The listing builds one solid part. Answer for the finished solid, in the listing's coordinates (mm). Coordinates: 2 decimals unless noted, no trailing zeros. Loops run counter-clockwise (first coordinate to the right, second up) from the corner with the lowest first, then second, coordinate; pieces in that order, holes last. Notation, with made-up numbers: (-38.75, 50) - (9.25, 50) arc R23 cw to (9.25, 89) - close; hole circle Ø6 at (42.5, 43). An arc over 180 degrees is marked (long way). Put each result on its own line as item: value.
```python
from build123d import *

# Parameters (mm, degrees)
F0_R     = 6.35
F0_R_2   = 3.81
F1_DEPTH = 7.62


with BuildPart() as f1:
    # F0 (on Front) → F1 (new body)
    with BuildSketch(Plane.XZ):
        with BuildLine():
            ThreePointArc((-8.547501, -17.972921), (0, -26.520421), (8.547501, -17.972921))
            Line((8.547501, -17.972921), (5.813845, 25.207079))
            ThreePointArc((5.813845, 25.207079), (0, 31.020925), (-5.813845, 25.207079))
            Line((-5.813845, 25.207079), (-8.547501, -17.972921))
        make_face()
        with Locations((0, -17.972921)):
            Circle(F0_R, mode=Mode.SUBTRACT)
        with Locations((0, 25.207079)):
            Circle(F0_R_2, mode=Mode.SUBTRACT)
    extrude(amount=F1_DEPTH)


solid = f1.part
```
1) For a pull along X with two mould halves and no side action, classify faces 1 (the face through (0, -7.62, 3)), 2 (the face through (7.2, -3.8, 3.3)), 3 (the face through (-1.38, -3.76, -24.17)), 4 (the face through (-0.83, -3.76, 21.49)) as pulls with the +X half, pulls with the -X half, needs draft (parallel to the pull), parting line crosses it, or undercut.
Found:
face 1: needs draft
face 2: pulls with the +X half
face 3: undercut
face 4: undercut
2) Each of these flat-tipped pins is pushed along its axis until it touches: pin 1 (1 mm diameter, centred on y = -3, z = 10.5, fed in from -X); pin 2 (3 mm diameter, centred on y = -5.5, z = -2.5, fed in from -X); pin 3 (1.5 mm diameter, centred on y = -2.5, z = -1.5, fed in from -X); pin 4 (4 mm diameter, centred on x = -5.5, z = -3.5, fed in from +Y). Where does it stop, or does it pass through?
Found:
pin 1: stops at x = -6.78
pin 2: stops at x = -7.66
pin 3: stops at x = -7.55
pin 4: stops at y = 0
3) The part is cut by section C-C (z = -16). Give the vertices of the cut face in (x, y), and give its area (3 significant figures).
Found:
outline: (-8.42, -7.62) - (-6.04, -7.62) - (-6.04, 0) - (-8.42, 0) - close; (6.04, -7.62) - (8.42, -7.62) - (8.42, 0) - (6.04, 0) - close
area: 36.4 mm^2
4) Straight lines are drawn through the part: L1, parallel to Z at x = 0, y = -2.75; L2, parallel to X at y = -4.5, z = -18; L3, parallel to Z at x = -2.5, y = -6.75. For each, find the intervals that lie inside material, in ascending order. Write a range as [from, to].
Found:
L1: z = [-26.52, -24.32], [-11.62, 21.4], [29.02, 31.02]
L2: x = [-8.55, -6.35], [6.35, 8.55]
L3: z = [-26.15, -23.81], [-12.14, 22.33], [28.08, 30.46]
5) The part is cut by section A-A (x = 0). Give the vertices of the cut face in (y, z).
Found:
outline: (-7.62, -26.52) - (0, -26.52) - (0, -24.32) - (-7.62, -24.32) - close; (-7.62, -11.62) - (0, -11.62) - (0, 21.4) - (-7.62, 21.4) - close; (-7.62, 29.02) - (0, 29.02) - (0, 31.02) - (-7.62, 31.02) - close
6) The part is cut by section D-D (z = 4.5). Give the vertices of the cut face in (x, y).
Found:
outline: (-7.12, -7.62) - (7.12, -7.62) - (7.12, 0) - (-7.12, 0) - close
7) The part is cut by section B-B (y = -6.75). State how many separate pieces and enclosed holes the cut face has, and give its area (3 significant figures).
Found:
separate pieces: 1
enclosed holes: 2
area: 616 mm^2
